CAD build for the part. Positions are in the model's coordinates, mm. A direction names the side the tool comes from. Coordinates: 2 decimals unless noted, no trailing zeros. Loops run counter-clockwise (first coordinate to the right, second up) from the corner with the lowest first, then second, coordinate; pieces in that order, holes last.
1) Two-plate mould, pull along Y, no slides. Class faces 1 (the flat face through (-21, 50, 0)), 2 (the flat face through (-5.493, 116.72, 15.21)), 3 (the cylindrical face through (-34.743, 71.753, 14.79)): +Y half, -Y half, draft (parallel to the pull), parting line (faces both ways), or undercut.
2) Pin check, flat tips, straight feed: pin 1 Ø4 at (x, y) = (-40, 5) entering from -Z; pin 2 Ø1.5 at (y, z) = (42.5, 11) entering from -X; pin 3 Ø5 at (y, z) = (71, 20) entering from -X; pin 4 Ø1.5 at (x, y) = (-20.5, 89.5) entering from +Z. Stop position of each tip, or through.
3) Saw through at B-B, the plane y = 65. Write the cut outline in (x, z), and give its area (3 significant figures).
4) Which spindle directions (+Z, -Z, +X, -X, +Y, -Y) get a long thin tool onto all of the face, cutting with end or side? Do faces 4 (the flat face through (-1.6, 36, 15)), 5 (the flat face through (-23, 0, 15)). Say none if no direction does.
5) Wall check: line 1 along X through (y, z) = (102, 22.25); line 2 along X through (y, z) = (40.5, 1.5); line 3 along X through (y, z) = (35.5, 3.75). Give the ranges that are in metal, low to high.
6) Saw through at C-C, the plane z = 4. Give the number of separate pieces and of enclosed holes in the cut face, and give its area (3 significant figures).
7) Saw through at A-A, the plane y = 129. Write the cut outline in (x, z).
```python
from build123d import *
from build123d.topology import SkipClean

# Parameters (mm, degrees)
BOSS_EXTRUDE4_DEPTH = 30
SKETCH12_R          = 1.65
CUT_EXTRUDE1_DEPTH  = 151.461734423
CUT_EXTRUDE2_START  = -20
CUT_EXTRUDE2_DEPTH  = 20
CUT_EXTRUDE3_START  = -30
CUT_EXTRUDE3_DEPTH  = 30
BOSS_EXTRUDE5_DEPTH = 30
CIRPATTERN1_COUNT   = 6
CIRPATTERN1_ANGLE   = 30
LPATTERN2_COUNT     = 3
LPATTERN2_PITCH     = 10
CUT_EXTRUDE4_START  = -30
CUT_EXTRUDE4_DEPTH  = 30
BOSS_EXTRUDE7_DEPTH = 30
LPATTERN3_COUNT     = 2
LPATTERN3_PITCH     = 16
CUT_EXTRUDE5_START  = -30
CUT_EXTRUDE5_DEPTH  = 30


with BuildPart() as part:
    # Sketch5 → Boss-Extrude4 (new body)
    with BuildSketch(Plane.XY):
        with BuildLine():
            Line((0, 0), (0, 138.405603612))
            ThreePointArc((0, 138.405603612), (-1.431938837, 140.323234054), (-3.677306515, 139.494934991))
            ThreePointArc((-3.677306515, 139.494934991), (-34.45212059, 72.743387818), (-45, 0))
            Line((-45, 0), (0, 0))
        make_face()
        with BuildLine():
            Line((-1.6, 10), (-40.801596678, 10))
            ThreePointArc((-40.801596678, 10), (-30.171322984, 73.09445494), (-4, 131.480881584))
            ThreePointArc((-4, 131.480881584), (-2.54422163, 132.052107892), (-1.6, 130.805498221))
            Line((-1.6, 130.805498221), (-1.6, 10))
        make_face(mode=Mode.SUBTRACT)
    extrude(amount=BOSS_EXTRUDE4_DEPTH)

    # Sketch12 → Cut-Extrude1 (cut, through all)
    with BuildSketch(Plane.XY.offset(30)):
        with Locations((-40, 5)):
            Circle(SKETCH12_R)
        with Locations((-22.5, 5)):
            Circle(SKETCH12_R)
        with Locations((-5, 5)):
            Circle(SKETCH12_R)
    extrude(amount=-CUT_EXTRUDE1_DEPTH, mode=Mode.SUBTRACT)

    # Sketch17 → Cut-Extrude2 (cut)
    with BuildSketch(Plane.XY.offset(30).offset(CUT_EXTRUDE2_START)):
        Polygon((-109.129206393, -31.174044695), (890.870793607, -18.386269912), (884.13367644, 508.454191469), (-120.638203698, 868.825955305), (-717.462714608, 272.001444394), align=None)
        with BuildLine():
            Line((-45, 0), (0, 0))
            Line((0, 0), (0, 138.405603612))
            ThreePointArc((0, 138.405603612), (-0.890765175, 140.069814567), (-2.769598102, 140.25160436))
            ThreePointArc((-2.769598102, 140.25160436), (-57.041683198, 80.109492203), (-45, 0))
        make_face(mode=Mode.SUBTRACT)
    extrude(amount=CUT_EXTRUDE2_DEPTH, mode=Mode.SUBTRACT)

    # Sketch18 → Cut-Extrude3 (cut)
    with BuildSketch(Plane.XY.offset(30).offset(CUT_EXTRUDE3_START)):
        Polygon((10.567687301, -7.152622061), (26.572035637, 318.782087337), (-234.729728554, 306.471050155), (-205.798791176, -46.855716973), align=None)
        with BuildLine():
            Line((-45, 0), (0, 0))
            Line((0, 0), (0, 138.405603612))
            ThreePointArc((0, 138.405603612), (-1.431938837, 140.323234054), (-3.677306515, 139.494934991))
            ThreePointArc((-3.677306515, 139.494934991), (-34.45212059, 72.743387818), (-45, 0))
        make_face(mode=Mode.SUBTRACT)
    extrude(amount=CUT_EXTRUDE3_DEPTH, mode=Mode.SUBTRACT)

    # Sketch14 → Boss-Extrude5 (add)
    with BuildSketch(Plane.XY.offset(30)):
        Polygon((48.4, 10), (-108.88130356, 76.761952422), (-108.099841303, 78.602962129), (49.181462257, 11.841009707), align=None)
    boss_extrude5 = extrude(amount=-BOSS_EXTRUDE5_DEPTH)

    # CirPattern1: Boss-Extrude5 ×6 about axis
    cirpattern1_axis = Axis((49.181462257, 11.841009707, 0), (0, 0, -1))
    for i in range(1, CIRPATTERN1_COUNT):
        add(boss_extrude5.rotate(cirpattern1_axis, i * CIRPATTERN1_ANGLE / (CIRPATTERN1_COUNT - 1)))

    # LPattern2: Boss-Extrude5 ×3
    with Locations(*[(0, -i * LPATTERN2_PITCH, 0) for i in range(1, LPATTERN2_COUNT)]):
        add(boss_extrude5)

    # Sketch20 → Cut-Extrude4 (cut)
    with BuildSketch(Plane.XY.offset(30).offset(CUT_EXTRUDE4_START)):
        Polygon((77.475806055, -29.017161833), (-265.551297842, 6.523481062), (-137.36538358, 367.52057294), (154.147754773, 113.145409747), align=None)
        with BuildLine():
            Line((-45, 0), (0, 0))
            Line((0, 0), (0, 138.405603612))
            ThreePointArc((0, 138.405603612), (-1.431938837, 140.323234054), (-3.677306515, 139.494934991))
            ThreePointArc((-3.677306515, 139.494934991), (-34.45212059, 72.743387818), (-45, 0))
        make_face(mode=Mode.SUBTRACT)
    extrude(amount=CUT_EXTRUDE4_DEPTH, mode=Mode.SUBTRACT)

    # Sketch21 → Boss-Extrude7 (add)
    with BuildSketch(Plane.XY.offset(30)):
        Polygon((-1.6, 92.230286229), (-0.00272898, 93.433916276), (-24.075329906, 125.379336678), (-25.672600926, 124.175706631), align=None)
    boss_extrude7 = extrude(amount=-BOSS_EXTRUDE7_DEPTH)

    # LPattern3: Boss-Extrude7 ×2
    with Locations(*[(0, i * LPATTERN3_PITCH, 0) for i in range(1, LPATTERN3_COUNT)]):
        add(boss_extrude7)

    # Sketch22 → Cut-Extrude5 (cut)
    with SkipClean():  # the faces are left unmerged after this step: merging them gives an invalid solid
        with BuildSketch(Plane.XY.offset(30).offset(CUT_EXTRUDE5_START)):
            Polygon((-56.498976092, -6.715699617), (29.926379711, -13.421115154), (17.260594809, 198.668694776), (-109.397254213, 188.734745833), align=None)
            with BuildLine():
                Line((0, 138.405603612), (0, 0))
                Line((0, 0), (-45, 0))
                ThreePointArc((-45, 0), (-34.45212059, 72.743387818), (-3.677306515, 139.494934991))
                ThreePointArc((-3.677306515, 139.494934991), (-1.431938837, 140.323234054), (0, 138.405603612))
            make_face(mode=Mode.SUBTRACT)
        extrude(amount=CUT_EXTRUDE5_DEPTH, mode=Mode.SUBTRACT)


solid = part.part
```
Data:
1. face 1: draft
1. face 2: undercut
1. face 3: +Y half
2. pin 1: stops at z = 0
2. pin 2: stops at x = -41.57
2. pin 3: stops at x = -35.67
2. pin 4: passes through
3. outline: (-36.61, 0) - (-32.48, 0) - (-32.48, 30) - (-36.61, 30) - close; (-30.22, 0) - (-26.74, 0) - (-26.74, 30) - (-30.22, 30) - close; (-15.02, 0) - (-11.97, 0) - (-11.97, 30) - (-15.02, 30) - close; (-3.12, 0) - (0, 0) - (0, 30) - (-3.12, 30) - close
3. area: 414 mm2
4. face 4: +Z, -Z
4. face 5: +Z, -Z, +X, -X, -Y
5. line 1: x = -23.81 to -18.76, -8.96 to -6.46, -1.6 to 0
5. line 2: x = -41.78 to -37.73, -23.45 to -18.33, -6.65 to -2.52, -1.6 to 0
5. line 3: x = -42.53 to -38.49, -35.23 to -30.11, -11.67 to -6.56, -1.6 to 0
6. separate pieces: 1
6. enclosed holes: 14
6. area: 1,840 mm2
7. outline: (-10.14, 0) - (-5.5, 0) - (-5.5, 30) - (-10.14, 30) - close; (-1.6, 0) - (0, 0) - (0, 30) - (-1.6, 30) - close
